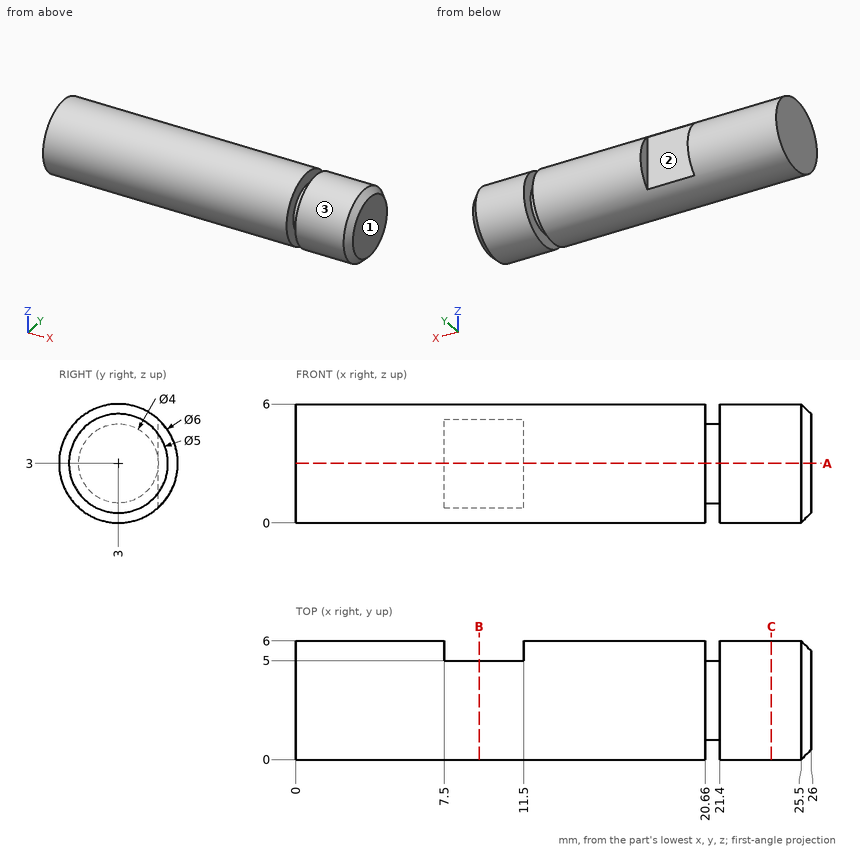
Study the drawing (mm; zero at the part's minimum x, y, z) and answer. Give positions to 0.01 mm unless a question says otherwise; leave off trailing zeros. Loops run counter-clockwise (first coordinate to the right, second up) from the corner with the lowest first, then second, coordinate; pieces in that order, holes last. Notation, with made-up numbers: (71.5, 39.5) - (85.5, 39.5) arc R19 ccw to (85.5, 67.5) - close; hole circle Ø11 at (28.25, 83). An arc over 180 degrees is marked (long way). Answer in a Markdown table with one row per item. Add a question column.
Q1. The part is cut by section A-A (z = 3). Determine the outline of the cut face in (x, y), and give its area (3 significant figures).
Q2. The part is cut by section B-B (x = 9.25). Determine the outline of the cut face in (y, z).
Q3. Determine the mould class of the marked faces 1, 2 and 3 for opening direction X: released by +X, released by -X, zero draft, split by the parting line, or undercut.
Q4. Each of these flat-tipped pins is pushed along its axis until it touches: P1, Ø1.8, axis at y = 2.5, z = 2.5, coming from the -X side; P2, Ø2, axis at x = 8.5, z = 4.5, coming from the -Y side. Where does it stop, or does it pass through?
Q5. The part is cut by section C-C (x = 24). Determine the outline of the cut face in (y, z).
Q6. Consider line 1 along X through (y, z) = (5.15, 4.1); line 2 along X through (y, z) = (3.7, 1); line 3 along X through (y, z) = (5.85, 2.7). Determine where each line is inside the solid, lowest interval first.
Solution:
| question | item | result |
|---|---|---|
| 1 | outline | (0, 0) - (20.66, 0) - (20.66, 1) - (21.4, 1) - (21.4, 0) - (25.5, 0) - (26, 0.5) - (26, 5.5) - (25.5, 6) - (21.4, 6) - (21.4, 5) - (20.66, 5) - (20.66, 6) - (11.5, 6) - (11.5, 5) - (7.5, 5) - (7.5, 6) - (0, 6) - close |
| 1 | area | 150 mm² |
| 2 | outline | (5, 0.76) - (5, 5.24) arc R3 ccw (long way) to start |
| 3 | face 1 | released by +X |
| 3 | face 2 | undercut |
| 3 | face 3 | zero draft |
| 4 | P1 | stops at x = 0 |
| 4 | P2 | stops at y = 0.04 |
| 5 | outline | circle Ø6 at (3, 3) |
| 6 | line 1 | x = 0 to 7.5, 11.5 to 20.66, 21.4 to 26 |
| 6 | line 2 | x = 0 to 20.66, 21.4 to 26 |
| 6 | line 3 | x = 0 to 7.5, 11.5 to 20.66, 21.4 to 25.63 |
